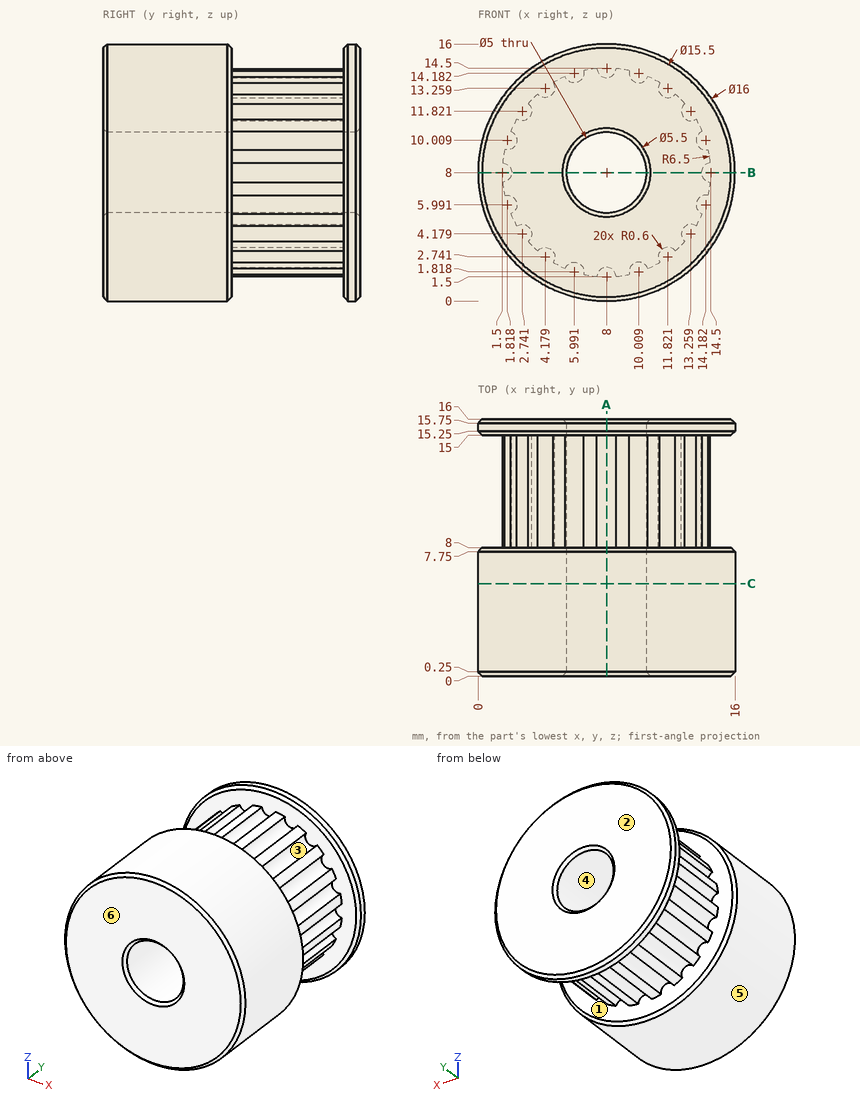
Check sheet for the drawn part. Datum: minimum x, y, z corner. Units: mm. A direction names the side the tool comes from. Coordinates: 2 decimals unless noted, no trailing zeros. Write each loop counter-clockwise with the first axis right and the second up, starting at its lowest first coordinate (ties: lowest second). Pieces come first, ordered by that corner, then holes. Notation, with made-up numbers: M -24.5,29.25 L 5.5,29.25 A9 cw 5.5,41.25 Z; hole C 19.25,-12.5 d3. An arc over 180 degrees is marked long. Use a Markdown table: item, result.
Q1. Sectioned sample at C-C, the plane y = 5.75. Record the boundary of the cut face in (x, z), plus the area to 3 significant figures.
Reply:
| item | result |
|---|---|
| outline | C 8,8 d16; hole C 8,8 d5 |
| area | 181 mm² |
Q2. Go/stop test with flat-tipped pins: P1, Ø1.5, axis at y = 4.5, z = 9, coming from the -X side; P2, Ø3, axis at y = 14, z = 13, coming from the +X side (1 decimal); P3, Ø3, axis at y = 8, z = 10.5, coming from the -X side (1 decimal). Record where each tip stops, or that it passes through.
Reply:
| item | result |
|---|---|
| P1 | stops at x = 0 |
| P2 | stops at x = 14.8 |
| P3 | stops at x = 0.1 |
Q3. Sectioned sample at A-A, the plane x = 8. Record the boundary of the cut face in (y, z).
Reply:
| item | result |
|---|---|
| outline | M 0,0.25 L 0.25,0 L 7.75,0 L 8,0.25 L 8,2.1 L 15,2.1 L 15,0.25 L 15.25,0 L 15.75,0 L 16,0.25 L 16,5.25 L 15.75,5.5 L 0.25,5.5 L 0,5.25 Z; M 0,10.75 L 0.25,10.5 L 15.75,10.5 L 16,10.75 L 16,15.75 L 15.75,16 L 15.25,16 L 15,15.75 L 15,13.9 L 8,13.9 L 8,15.75 L 7.75,16 L 0.25,16 L 0,15.75 Z |
Q4. Thickness scan on line 1 (Z direction, x = 8, y = 5.75); line 2 (Y direction, x = 14, z = 4.25); line 3 (Z direction, x = 8, y = 11.5). Record the ranges inside material, lowest first.
Reply:
| item | result |
|---|---|
| line 1 | z = 0 to 5.5, 10.5 to 16 |
| line 2 | y = 0 to 8, 15 to 16 |
| line 3 | z = 2.1 to 5.5, 10.5 to 13.9 |
Q5. Set-up check for the marked faces 1 and 2: record each of +Z, -Z, +X, -X, +Y, -Y from which the full face is reachable in a straight line by a thin tool's end or side.
Reply:
| item | result |
|---|---|
| face 1 | none |
| face 2 | +Z, -Z, +X, -X, +Y |
Q6. Draft check along X on the marked faces 3, 4, 5 and 6. Enter one of: +X half, -X half, draft (parallel to the pull), parting line (faces both ways), or undercut.
Reply:
| item | result |
|---|---|
| face 3 | undercut |
| face 4 | undercut |
| face 5 | parting line |
| face 6 | draft |
Q7. Sectioned sample at B-B, the plane z = 8. Record the boundary of the cut face in (x, y), plus the area to 3 significant figures.
Reply:
| item | result |
|---|---|
| outline | M 0,0.25 L 0.25,0 L 5.25,0 L 5.5,0.25 L 5.5,15.75 L 5.25,16 L 0.25,16 L 0,15.75 L 0,15.25 L 0.25,15 L 2.1,15 L 2.1,8 L 0.25,8 L 0,7.75 Z; M 10.5,0.25 L 10.75,0 L 15.75,0 L 16,0.25 L 16,7.75 L 15.75,8 L 13.9,8 L 13.9,15 L 15.75,15 L 16,15.25 L 16,15.75 L 15.75,16 L 10.75,16 L 10.5,15.75 Z |
| area | 146 mm² |
